```python
from build123d import *
from OCP.BRepFilletAPI import BRepFilletAPI_MakeChamfer

# Parameters (mm, degrees)
SKETCH1_W           = 8
SKETCH1_H           = 13
BOSS_EXTRUDE1_DEPTH = 9
SKETCH2_W           = 10
SKETCH2_H           = 15
BOSS_EXTRUDE2_DEPTH = 1.5
CHAMFER1_SIZE       = 1.2
CHAMFER1_SIZE2      = 1.430104311
SKETCH3_W           = 5.725577816
SKETCH3_H           = 10.725577816
BOSS_EXTRUDE3_DEPTH = 2.5
CUT_EXTRUDE2_DEPTH  = 10
CUT_EXTRUDE3_DEPTH  = 10
SKETCH6_W           = 4
SKETCH6_H           = 0.4
BOSS_EXTRUDE4_DEPTH = 5
CHAMFER2_SIZE       = 0.6
LPATTERN1_COUNT     = 2
LPATTERN1_PITCH     = 5
CHAMFER3_SIZE       = 0.6


with BuildPart() as part:
    # Sketch1 → Boss-Extrude1 (new body)
    with BuildSketch(Plane(origin=(0, 0, 0), x_dir=(1, 0, 0), z_dir=(0, 1, 0))):
        Rectangle(SKETCH1_W, SKETCH1_H)
    extrude(amount=BOSS_EXTRUDE1_DEPTH)

    # Sketch2 → Boss-Extrude2 (add)
    with BuildSketch(Plane(origin=(0, 9, 0), x_dir=(1, 0, 0), z_dir=(0, 1, 0))):
        Rectangle(SKETCH2_W, SKETCH2_H)
    extrude(amount=BOSS_EXTRUDE2_DEPTH)

    # Chamfer1: one chamfer whose edges measure the first distance from different faces: ONE call of the kernel's chamfer builder (chamfer() names one face for all edges)
    chamfer1_edges_1 = [part.edges().sort_by_distance(p)[0] for p in [
        (5, 10.5, 0),
    ]]
    chamfer1_side_1 = [part.faces().sort_by_distance(p)[0] for p in [
        (5, 9.75, 0),
    ]]
    chamfer1_edges_2 = [part.edges().sort_by_distance(p)[0] for p in [
        (0, 10.5, -7.5),
    ]]
    chamfer1_side_2 = [part.faces().sort_by_distance(p)[0] for p in [
        (0, 9.75, -7.5),
    ]]
    chamfer1_edges_3 = [part.edges().sort_by_distance(p)[0] for p in [
        (-5, 10.5, 0),
    ]]
    chamfer1_side_3 = [part.faces().sort_by_distance(p)[0] for p in [
        (-5, 9.75, 0),
    ]]
    chamfer1_edges_4 = [part.edges().sort_by_distance(p)[0] for p in [
        (0, 10.5, 7.5),
    ]]
    chamfer1_side_4 = [part.faces().sort_by_distance(p)[0] for p in [
        (0, 9.75, 7.5),
    ]]
    chamfer1 = BRepFilletAPI_MakeChamfer(part.part.solid().wrapped)
    for e in chamfer1_edges_1:
        chamfer1.Add(CHAMFER1_SIZE, CHAMFER1_SIZE2, e.wrapped, chamfer1_side_1[0].wrapped)  # the first distance lies on this face
    for e in chamfer1_edges_2:
        chamfer1.Add(CHAMFER1_SIZE, CHAMFER1_SIZE2, e.wrapped, chamfer1_side_2[0].wrapped)  # the first distance lies on this face
    for e in chamfer1_edges_3:
        chamfer1.Add(CHAMFER1_SIZE, CHAMFER1_SIZE2, e.wrapped, chamfer1_side_3[0].wrapped)  # the first distance lies on this face
    for e in chamfer1_edges_4:
        chamfer1.Add(CHAMFER1_SIZE, CHAMFER1_SIZE2, e.wrapped, chamfer1_side_4[0].wrapped)  # the first distance lies on this face
    add(Compound.cast(chamfer1.Shape()), mode=Mode.REPLACE)

    # Sketch3 → Boss-Extrude3 (add)
    with BuildSketch(Plane(origin=(0, 10.5, 0), x_dir=(1, 0, 0), z_dir=(0, 1, 0))):
        Rectangle(SKETCH3_W, SKETCH3_H)
    extrude(amount=BOSS_EXTRUDE3_DEPTH)

    # Sketch4 → Cut-Extrude2 (cut)
    with BuildSketch(Plane.ZY.offset(2.862788908)):
        Polygon((5.362788908, 13), (3.862788908, 13), (5.362788908, 10.5), align=None)
    extrude(amount=-CUT_EXTRUDE2_DEPTH, mode=Mode.SUBTRACT)

    # Sketch5 → Cut-Extrude3 (cut)
    with BuildSketch(Plane.ZY.offset(2.862788908)):
        with BuildLine():
            Line((-5.362788908, 10.5), (-5.362788908, 13))
            Line((-5.362788908, 13), (3.862788908, 13))
            add(Edge.make_bspline(
                [(3.862788908, 13), (-0.886352769, 10.585649202), (-5.362788908, 10.5)],
                knots=[0, 0, 0, 0.869788285, 0.869788285, 0.869788285], degree=2))
        make_face()
    extrude(amount=-CUT_EXTRUDE3_DEPTH, mode=Mode.SUBTRACT)

    # Sketch6 → Boss-Extrude4 (add)
    with BuildSketch(Plane.XZ):
        with Locations((0, 5)):
            Rectangle(SKETCH6_W, SKETCH6_H)
    boss_extrude4 = extrude(amount=BOSS_EXTRUDE4_DEPTH)

    # Chamfer2
    chamfer2_edges = [part.edges().sort_by_distance(p)[0] for p in [
        (2, -5, 5),
        (-2, -5, 5),
    ]]
    chamfer(chamfer2_edges, length=CHAMFER2_SIZE)

    # LPattern1: Boss-Extrude4 ×2
    with Locations(*[(0, 0, -i * LPATTERN1_PITCH) for i in range(1, LPATTERN1_COUNT)]):
        add(boss_extrude4)

    # Chamfer3
    chamfer3_edges = [part.edges().sort_by_distance(p)[0] for p in [
        (2, -5, 0),
        (-2, -5, 0),
    ]]
    chamfer(chamfer3_edges, length=CHAMFER3_SIZE)


solid = part.part
```
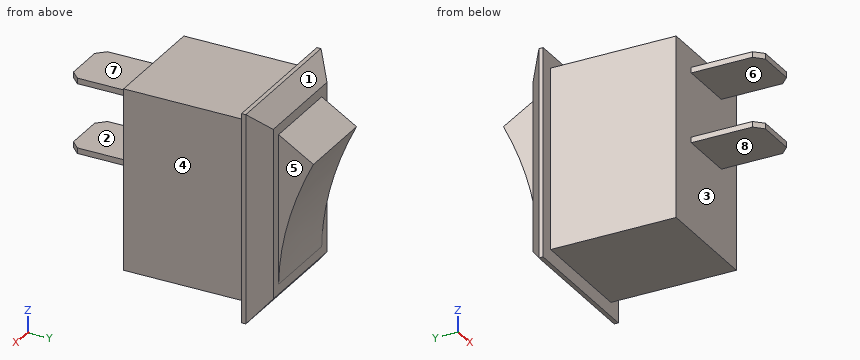
Work out the finished part from the listing and answer in its coordinate system (mm). Face numbers are marked on the shaded views. A direction names the side the tool comes from. Give positions to 0.01 mm unless a question says otherwise; leave off trailing zeros. Loops run counter-clockwise (first coordinate to the right, second up) from the corner with the lowest first, then second, coordinate; pieces in that order, holes last. Notation, with made-up numbers: (11.5, -12.5) - (54.5, -12.5) arc R18 ccw to (54.5, 7.5) - close; hole circle Ø8 at (86, -22.75). An arc over 180 degrees is marked (long way). Use CSV: the item, a comma, the result in double quotes. Start each with the question number.
(1) Find section C-C, the plane y = 5.75. Determine the outline of the cut face in (x, z), plus the area to 3 significant figures.
(2) Find the intervals of material crossed by L1, parallel to Y at x = 3.5, z = 4.25; L2, parallel to Z at x = 0, y = 1.5; L3, parallel to X at y = 6.75, z = -3.25, in increasing order.
(3) A tool of negligible diameter and unlimited length cuts with its end or side. For the marked faces 5, 6, 7 and 8, from which of +Z, -Z, +X, -X, +Y, -Y can it reach the whole face along a straight path? Write none if from no direction.
(4) Determine the mould class of the marked faces 1, 2, 3 and 4 for opening direction Z: released by +Z, released by -Z, zero draft, split by the parting line, or undercut.
(5) Find section B-B, the plane x = 4.25. Determine the outline of the cut face in (y, z), plus the area to 3 significant figures.
(6) Each of these flat-tipped pins is pushed along its axis until it touches: pin 1 (1.5 mm diameter, centred on x = -1, z = 4, fed in from +Y); pin 2 (1.5 mm diameter, centred on x = 1.5, z = -5, fed in from +Y); pin 3 (1.5 mm diameter, centred on x = -0.5, z = -3.5, fed in from +Y); pin 4 (4.5 mm diameter, centred on x = -1, y = -2.5, fed in from +Z). Where does it stop, or does it pass through?
(7) Find section A-A, the plane y = -3.5. Determine the outline of the cut face in (x, z), plus the area to 3 significant figures.
Results found:
1,outline,"(-4, -6.5) - (4, -6.5) - (4, 6.5) - (-4, 6.5) - close"
1,area,"104 mm^2"
2,L1,"0 to 10.5"
2,L2,"-6.5 to 6.5"
2,L3,"-4 to 4"
3,face 5,"+Z, -Z, +X, +Y"
3,face 6,"+X, -X, -Y"
3,face 7,"+Z, +X, -X, -Y"
3,face 8,"-Z, +X, -X, -Y"
4,face 1,"released by +Z"
4,face 2,"undercut"
4,face 3,"undercut"
4,face 4,"zero draft"
5,outline,"(9, -7.5) - (9.3, -7.5) - (9.93, -6.75) - (9.93, 6.75) - (9.3, 7.5) - (9, 7.5) - close"
5,area,"13.5 mm^2"
6,pin 1,"y = 13"
6,pin 2,"y = 10.56"
6,pin 3,"y = 10.74"
6,pin 4,"z = 5.2"
7,outline,"(-2, -0.2) - (2, -0.2) - (2, 0.2) - (-2, 0.2) - close; (-2, 4.8) - (2, 4.8) - (2, 5.2) - (-2, 5.2) - close"
7,area,"3.20 mm^2"
